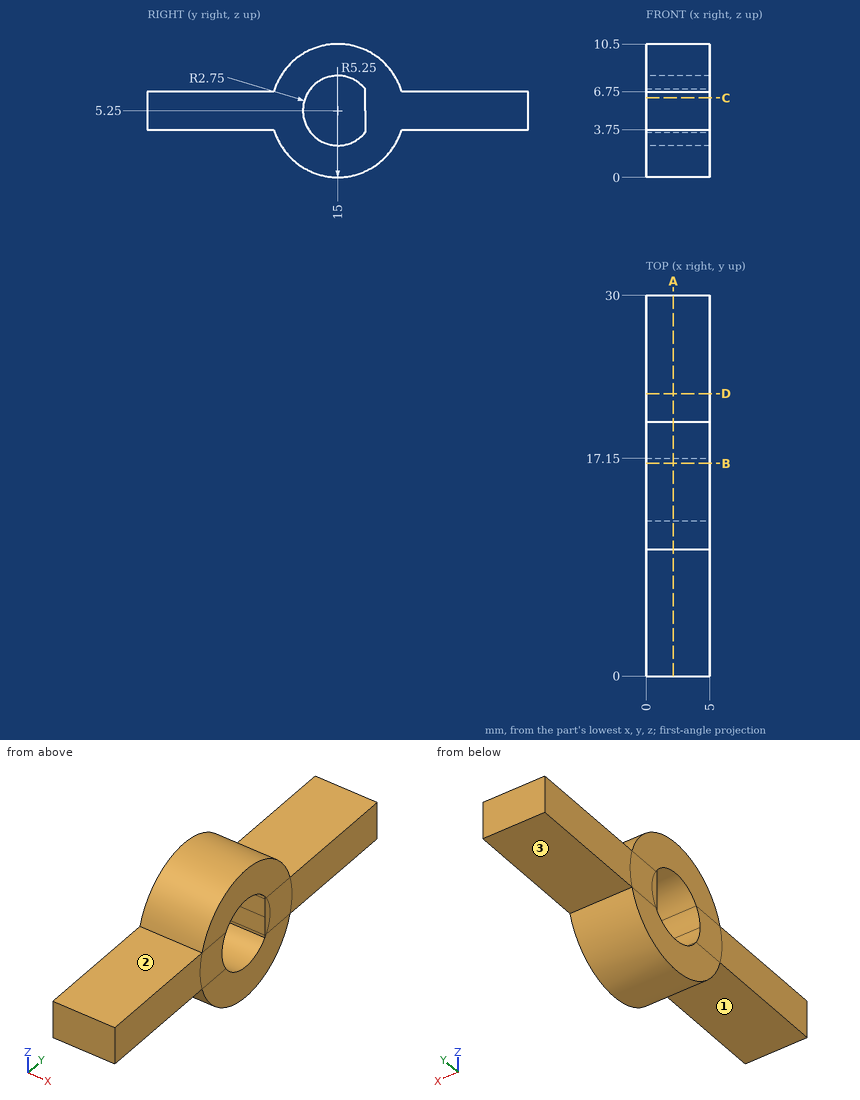
Here's the drawing with two shaded views (mm, measured from the low corner). I have some questions. A direction names the side the tool comes from. Coordinates: 2 decimals unless noted, no trailing zeros. Write each loop counter-clockwise with the first axis right and the second up, starting at its lowest first coordinate (ties: lowest second). Pieces come first, ordered by that corner, then holes.
Item 1: I want a section at C-C on z = 6.25. Write out the boundary of the cut face in (x, y), and give its area (3 significant figures).
Item 2: I want a section at A-A on x = 2.15. Write out the boundary of the cut face in (y, z), and give its area (3 significant figures).
Item 3: If I drill on line 1 (Y direction, x = 4.4, z = 5.25); line 2 (Z direction, x = 1.05, y = 25.25); line 3 (Y direction, x = 0.85, z = 3), over which ranges is the centre line in solid material (lowest first)?
Item 4: I want a section at B-B on y = 16.75. Write out the boundary of the cut face in (x, z).
Item 5: I want a section at D-D on y = 22.25. Write out the boundary of the cut face in (x, z), and give its area (3 significant figures).
Item 6: On a 3-axis mill with a long thin cutter (end or side, diameter ignored), from which of +Z, -Z, +X, -X, +Y, -Y can I reach the whole of each face in a straight line? I mean the marked faces 1, 2 and 3. Say none if no direction works.
Item 7: Will these pins go through, and if not, where does the flat tip stop? pin 1 (2.5 mm diameter, centred on x = 1.5, y = 2.5, fed in from +Z); pin 2 (2.5 mm diameter, centred on x = 3, y = 5.5, fed in from -Z).
Findings below:
1. outline: (0, 0) - (5, 0) - (5, 12.44) - (0, 12.44) - close; (0, 17.15) - (5, 17.15) - (5, 30) - (0, 30) - close
1. area: 126 mm2
2. outline: (0, 3.75) - (9.97, 3.75) arc R5.25 ccw to (20.03, 3.75) - (30, 3.75) - (30, 6.75) - (20.03, 6.75) arc R5.25 ccw to (9.97, 6.75) - (0, 6.75) - close; hole (17.15, 3.54) - (17.15, 6.96) arc R2.75 ccw (long way) to start
2. area: 123 mm2
3. line 1: y = 0 to 12.25, 17.15 to 30
3. line 2: z = 3.75 to 6.75
3. line 3: y = 10.26 to 13.42, 16.58 to 19.74
4. outline: (0, 0.3) - (5, 0.3) - (5, 3.13) - (0, 3.13) - close; (0, 7.37) - (5, 7.37) - (5, 10.2) - (0, 10.2) - close
5. outline: (0, 3.75) - (5, 3.75) - (5, 6.75) - (0, 6.75) - close
5. area: 15.0 mm2
6. face 1: -Z, +X, -X, -Y
6. face 2: +Z, +X, -X, -Y
6. face 3: -Z, +X, -X, +Y
7. pin 1: stops at z = 6.75
7. pin 2: stops at z = 3.75
